Source: CAD feature listing. Evaluate the final solid. Frame: model axes, mm. Give positions to 0.01 mm unless a question says otherwise; leave off trailing zeros. Order: outer loops, then holes, each group sorted by start corner. A loop starts at its lowest first (then second) coordinate and runs counter-clockwise, first axis right, second up. Notation, with made-up numbers: M 43.5,54.25 L 92.5,54.25 A9 ccw 92.5,58.25 Z; hole C 85,9.5 d11. An arc over 180 degrees is marked long. Use CSV: the item, a comma, the result in double quotes. Start each with the question number.
Item 1: Ray query, probe 1 along X at (y, z) = (-67, -0.4); probe 2 along Y at (x, z) = (-59.5, -1.8); probe 3 along X at (y, z) = (51, -2.95). Return the intervals inside material, ascending. Write a range as from..to.
Item 2: Pull-direction query (Y, two-part tool) for faces 1 (the face through (41.116, 97.255, -1.61)), 2 (the face through (-45.549, 97.255, -1.61)), 3 (the face through (-1, 2, -3.175)); classes: +Y half, -Y half, draft (parallel to the pull), parting line (faces both ways), or undercut.
Item 3: First-contact query: pin 1 (4 mm diameter, centred on x = 59.69, y = 52.51, fed in from -Z); pin 2 (6 mm diameter, centred on x = 43.33, y = 96.96, fed in from -Z) (3 decimals). Flat tips, straight axial feed; report the tip coordinate or a pass-through.
Item 4: Section query C-C on z = -1.25. Count the separate pieces of the cut face and the enclosed holes in it, and give its area (3 significant figures).
Item 5: Section query B-B on y = -68. Return loops of the section in (x, z) (3 decimals).
Item 6: Section query A-A on x = 31.75. Return loops of the section in (y, z) (1 decimal), and give its area (3 significant figures).
Autodesk Inventor part; units mm, degrees
ref_plane "YZ Plane" through (0, 0, 0) normal (1, 0, 0) x (0, 1, 0)
ref_plane "XZ Plane" through (0, 0, 0) normal (0, 1, 0) x (-1, 0, 0)
ref_plane "XY Plane" through (0, 0, 0) normal (0, 0, 1) x (1, 0, 0)
sketch "Sketch1" plane through (0, 0, 0) normal (0, 0, 1) x (1, 0, 0)
  line L0 (-68.58, -128.7145) -> (68.58, -128.7145)
  line L1 (68.58, -128.7145) -> (68.58, 128.7145)
  line L2 (68.58, 128.7145) -> (-68.58, 128.7145)
  line L3 (-68.58, 128.7145) -> (-68.58, -128.7145)
  line L4 (-68.58, -128.7145) -> (68.58, 128.7145) construction
  line L5 (68.58, -128.7145) -> (-68.58, 128.7145) construction
  point P0 (0, 0)
  dimension "d0" = 137.16
  dimension "d1" = 257.429
extrude "Extrusion1" add sketch "Sketch1" against normal blind 3.175
sketch "Sketch2" plane through (0, 0, 0) normal (0, 0, 1) x (1, 0, 0)
  circle A0 centre (-59.69, 52.5145) radius 2.0955
  line L0 (-68.58, 128.7145) -> (-68.58, -128.7145)
  line L1 (-68.58, 128.7145) -> (68.58, 128.7145)
  circle A1 centre (59.69, 52.5145) radius 2.0955
  line L2 (68.58, -128.7145) -> (68.58, 128.7145)
  circle A2 centre (-59.69, -116.0145) radius 2.0955
  circle A3 centre (59.69, -116.0145) radius 2.0955
  line L3 (-68.58, -128.7145) -> (68.58, -128.7145)
  point P0 (0, 0)
  dimension "d4" = 8.89
  dimension "d5" = 76.2
  dimension "d6" = 76.2
  dimension "d7" = 8.89
  dimension "d8" = 4.191
  dimension "d9" = 12.7
  dimension "d10" = 8.89
  dimension "d11" = 8.89
  dimension "d12" = 12.7
  dimension "d13" = 4.191
  dimension "d21" = 4.191
  dimension "d22" = 4.191
hole "Hole1" at (-59.69, 52.5145, 0) at (59.69, 52.5145, 0) at (-59.69, -116.0145, 0) at (59.69, -116.0145, 0) direction (0, 0, -1) diameter 4.191 end through all
sketch "Sketch4" plane through (0, 0, 0) normal (0, 0, 1) x (1, 0, 0)
  line L0 (-35.179, -49.0855) -> (-35.179, -99.8855)
  line L1 (-28.321, -49.0855) -> (-28.321, -99.8855)
  line L2 (28.321, -49.0855) -> (28.321, -99.8855)
  line L3 (35.179, -49.0855) -> (35.179, -99.8855)
  line L4 (-68.58, 128.7145) -> (-68.58, -128.7145)
  line L5 (68.58, -128.7145) -> (68.58, 128.7145)
  line L6 (-68.58, -128.7145) -> (68.58, -128.7145)
  arc A0 (-28.321, -49.0855) -> (-35.179, -49.0855) centre (-31.75, -49.0855) ccw
  arc A1 (-35.179, -99.8855) -> (-28.321, -99.8855) centre (-31.75, -99.8855) ccw
  arc A2 (35.179, -49.0855) -> (28.321, -49.0855) centre (31.75, -49.0855) ccw
  arc A3 (28.321, -99.8855) -> (35.179, -99.8855) centre (31.75, -99.8855) ccw
  point P0 (0, 0)
  dimension "d23" = 6.858
  dimension "d24" = 6.858
  dimension "d25" = 33.401
  dimension "d26" = 50.8
  dimension "d27" = 33.401
  dimension "d28" = 28.829
  dimension "d29" = 28.829
  dimension "d30" = 28.829
  dimension "d31" = 28.829
  dimension "d32" = 50.8
  dimension "d33" = 50.8
  dimension "d34" = 50.8
extrude "Extrusion2" cut sketch "Sketch4" against normal blind 3.175
sketch "Sketch5" plane through (0, 0, 0) normal (0, 0, 1) x (1, 0, 0)
  line L0 (-68.58, 128.7145) -> (68.58, 128.7145)
  line L1 (68.58, 128.7145) -> (68.58, -128.7145)
  point P0 (0, 0)
  point P1 (-43.3324, 96.9645)
  point P2 (43.3324, 96.9645)
  dimension "d37" = 31.75
  dimension "d38" = 86.6648
  dimension "d39" = 31.75
  dimension "d40" = 25.2476
hole "Hole2" at (-43.3324, 96.9645, 0) at (43.3324, 96.9645, 0) direction (0, 0, -1) diameter 4.4704 end through all
sketch "smartsensorPowered" plane through (0, 0, 0) normal (0, 0, 1) x (1, 0, 0)
  line L0 (-68.58, 128.7145) -> (-68.58, -128.7145)
  line L1 (68.58, 128.7145) -> (-68.58, 128.7145)
  line L2 (68.58, -128.7145) -> (68.58, 128.7145)
  line L3 (-44.45, 33.4645) -> (-16.51, 33.4645)
  line L4 (-16.51, 33.4645) -> (-16.51, -26.2255)
  line L5 (-16.51, -26.2255) -> (-44.45, -26.2255)
  line L6 (-44.45, -26.2255) -> (-44.45, 33.4645)
  circle A0 centre (-41.275, 30.2895) radius 1.651
  circle A1 centre (-40.64, -22.4155) radius 1.651
  circle A2 centre (-19.685, 2.9845) radius 1.651
  circle A3 centre (-19.685, 30.2895) radius 1.651
  line L7 (-3.81, 33.4645) -> (24.13, 33.4645)
  line L8 (24.13, 33.4645) -> (24.13, -26.2255)
  line L9 (24.13, -26.2255) -> (-3.81, -26.2255)
  line L10 (-3.81, -26.2255) -> (-3.81, 33.4645)
  circle A4 centre (-0.635, 30.2895) radius 1.651
  circle A5 centre (0, -22.4155) radius 1.651
  circle A6 centre (20.955, 2.9845) radius 1.651
  circle A7 centre (20.955, 30.2895) radius 1.651
  point P0 (0, 0)
  dimension "d52" = 27.94
  dimension "d53" = 59.69
  dimension "d59" = 3.175
  dimension "d60" = 3.175
  dimension "d61" = 3.302
  dimension "d62" = 3.302
  dimension "d63" = 3.175
  dimension "d64" = 3.175
  dimension "d66" = 3.81
  dimension "d67" = 3.81
  dimension "d68" = 3.302
  dimension "d69" = 30.48
  dimension "d70" = 3.175
  dimension "d71" = 3.302
  dimension "d72" = 27.94
  dimension "d73" = 59.69
  dimension "d74" = 3.175
  dimension "d75" = 3.175
  dimension "d76" = 3.302
  dimension "d77" = 3.302
  dimension "d78" = 3.175
  dimension "d79" = 3.175
  dimension "d80" = 3.81
  dimension "d81" = 3.81
  dimension "d82" = 3.302
  dimension "d83" = 30.48
  dimension "d84" = 3.175
  dimension "d85" = 3.302
  dimension "d86" = 12.7
sketch "BoardArea" plane through (0, 0, 0) normal (0, 0, 1) x (1, 0, 0)
  line L0 (-50.8, 39.8145) -> (50.8, 39.8145)
  line L1 (50.8, 39.8145) -> (50.8, -36.3855)
  line L2 (50.8, -36.3855) -> (-50.8, -36.3855)
  line L3 (-50.8, -36.3855) -> (-50.8, 39.8145)
  point P0 (0, 0)
sketch "teamflag" plane through (0, 0, 0) normal (0, 0, 1) x (1, 0, 0)
  line L0 (-3.81, -7.1755) -> (-44.45, -7.1755)
  line L1 (-44.45, -7.1755) -> (-44.45, 33.4645)
  line L2 (-44.45, 33.4645) -> (-3.81, 33.4645)
  line L3 (-3.81, 33.4645) -> (-3.81, -7.1755)
  circle A0 centre (-6.35, 30.9245) radius 1.651
  circle A1 centre (-41.91, 30.9245) radius 1.651
  circle A2 centre (-41.91, -4.6355) radius 1.651
  circle A3 centre (-6.35, -4.6355) radius 1.651
  line L4 (-50.8, -36.3855) -> (-50.8, 39.8145)
  circle A4 centre (-43.3324, 96.9645) radius 2.2352
  circle A5 centre (43.3324, 96.9645) radius 2.2352
  arc A6 (-35.179, -99.8855) -> (-28.321, -99.8855) centre (-31.75, -99.8855) ccw
  line L5 (-28.321, -99.8855) -> (-28.321, -49.0855)
  arc A7 (-28.321, -49.0855) -> (-35.179, -49.0855) centre (-31.75, -49.0855) ccw
  line L6 (-35.179, -49.0855) -> (-35.179, -99.8855)
  arc A8 (28.321, -99.8855) -> (35.179, -99.8855) centre (31.75, -99.8855) ccw
  line L7 (35.179, -99.8855) -> (35.179, -49.0855)
  arc A9 (35.179, -49.0855) -> (28.321, -49.0855) centre (31.75, -49.0855) ccw
  line L8 (28.321, -49.0855) -> (28.321, -99.8855)
  circle A10 centre (-59.69, -116.0145) radius 2.0955
  circle A11 centre (-59.69, 52.5145) radius 2.0955
  circle A12 centre (59.69, 52.5145) radius 2.0955
  circle A13 centre (59.69, -116.0145) radius 2.0955
  line L9 (68.58, 128.7145) -> (68.58, -128.7145)
  line L10 (68.58, -128.7145) -> (-68.58, -128.7145)
  line L11 (-68.58, -128.7145) -> (-68.58, 128.7145)
  line L12 (-68.58, 128.7145) -> (68.58, 128.7145)
  circle A14 centre (-43.3324, 96.9645) radius 2.2352
  circle A15 centre (43.3324, 96.9645) radius 2.2352
  arc A16 (-35.179, -99.8855) -> (-28.321, -99.8855) centre (-31.75, -99.8855) ccw
  line L13 (-28.321, -99.8855) -> (-28.321, -49.0855)
  arc A17 (-28.321, -49.0855) -> (-35.179, -49.0855) centre (-31.75, -49.0855) ccw
  line L14 (-35.179, -49.0855) -> (-35.179, -99.8855)
  arc A18 (28.321, -99.8855) -> (35.179, -99.8855) centre (31.75, -99.8855) ccw
  line L15 (35.179, -99.8855) -> (35.179, -49.0855)
  arc A19 (35.179, -49.0855) -> (28.321, -49.0855) centre (31.75, -49.0855) ccw
  line L16 (28.321, -49.0855) -> (28.321, -99.8855)
  circle A20 centre (-59.69, -116.0145) radius 2.0955
  circle A21 centre (-59.69, 52.5145) radius 2.0955
  circle A22 centre (59.69, 52.5145) radius 2.0955
  circle A23 centre (59.69, -116.0145) radius 2.0955
  line L17 (68.58, 128.7145) -> (68.58, -128.7145)
  line L18 (68.58, -128.7145) -> (-68.58, -128.7145)
  line L19 (-68.58, -128.7145) -> (-68.58, 128.7145)
  line L20 (-68.58, 128.7145) -> (68.58, 128.7145)
  circle A24 centre (-43.3324, 96.9645) radius 2.2352
  circle A25 centre (43.3324, 96.9645) radius 2.2352
  arc A26 (-35.179, -99.8855) -> (-28.321, -99.8855) centre (-31.75, -99.8855) ccw
  line L21 (-28.321, -99.8855) -> (-28.321, -49.0855)
  arc A27 (-28.321, -49.0855) -> (-35.179, -49.0855) centre (-31.75, -49.0855) ccw
  line L22 (-35.179, -49.0855) -> (-35.179, -99.8855)
  arc A28 (28.321, -99.8855) -> (35.179, -99.8855) centre (31.75, -99.8855) ccw
  line L23 (35.179, -99.8855) -> (35.179, -49.0855)
  arc A29 (35.179, -49.0855) -> (28.321, -49.0855) centre (31.75, -49.0855) ccw
  line L24 (28.321, -49.0855) -> (28.321, -99.8855)
  circle A30 centre (-59.69, -116.0145) radius 2.0955
  circle A31 centre (-59.69, 52.5145) radius 2.0955
  circle A32 centre (59.69, 52.5145) radius 2.0955
  circle A33 centre (59.69, -116.0145) radius 2.0955
  line L25 (68.58, 128.7145) -> (68.58, -128.7145)
  line L26 (68.58, -128.7145) -> (-68.58, -128.7145)
  line L27 (-68.58, -128.7145) -> (-68.58, 128.7145)
  line L28 (-68.58, 128.7145) -> (68.58, 128.7145)
  circle A34 centre (-43.3324, 96.9645) radius 2.2352
  circle A35 centre (43.3324, 96.9645) radius 2.2352
  arc A36 (-35.179, -99.8855) -> (-28.321, -99.8855) centre (-31.75, -99.8855) ccw
  line L29 (-28.321, -99.8855) -> (-28.321, -49.0855)
  arc A37 (-28.321, -49.0855) -> (-35.179, -49.0855) centre (-31.75, -49.0855) ccw
  line L30 (-35.179, -49.0855) -> (-35.179, -99.8855)
  arc A38 (28.321, -99.8855) -> (35.179, -99.8855) centre (31.75, -99.8855) ccw
  line L31 (35.179, -99.8855) -> (35.179, -49.0855)
  arc A39 (35.179, -49.0855) -> (28.321, -49.0855) centre (31.75, -49.0855) ccw
  line L32 (28.321, -49.0855) -> (28.321, -99.8855)
  circle A40 centre (-59.69, -116.0145) radius 2.0955
  circle A41 centre (-59.69, 52.5145) radius 2.0955
  circle A42 centre (59.69, 52.5145) radius 2.0955
  circle A43 centre (59.69, -116.0145) radius 2.0955
  line L33 (68.58, 128.7145) -> (68.58, -128.7145)
  line L34 (68.58, -128.7145) -> (-68.58, -128.7145)
  line L35 (-68.58, -128.7145) -> (-68.58, 128.7145)
  line L36 (-68.58, 128.7145) -> (68.58, 128.7145)
  circle A44 centre (-43.3324, 96.9645) radius 2.2352
  circle A45 centre (43.3324, 96.9645) radius 2.2352
  arc A46 (-35.179, -99.8855) -> (-28.321, -99.8855) centre (-31.75, -99.8855) ccw
  line L37 (-28.321, -99.8855) -> (-28.321, -49.0855)
  arc A47 (-28.321, -49.0855) -> (-35.179, -49.0855) centre (-31.75, -49.0855) ccw
  line L38 (-35.179, -49.0855) -> (-35.179, -99.8855)
  arc A48 (28.321, -99.8855) -> (35.179, -99.8855) centre (31.75, -99.8855) ccw
  line L39 (35.179, -99.8855) -> (35.179, -49.0855)
  arc A49 (35.179, -49.0855) -> (28.321, -49.0855) centre (31.75, -49.0855) ccw
  line L40 (28.321, -49.0855) -> (28.321, -99.8855)
  circle A50 centre (-59.69, -116.0145) radius 2.0955
  circle A51 centre (-59.69, 52.5145) radius 2.0955
  circle A52 centre (59.69, 52.5145) radius 2.0955
  circle A53 centre (59.69, -116.0145) radius 2.0955
  line L41 (68.58, 128.7145) -> (68.58, -128.7145)
  line L42 (68.58, -128.7145) -> (-68.58, -128.7145)
  line L43 (-68.58, -128.7145) -> (-68.58, 128.7145)
  line L44 (-68.58, 128.7145) -> (68.58, 128.7145)
  line L45 (-50.8, 39.8145) -> (50.8, 39.8145)
  line L46 (43.18, -7.1755) -> (2.54, -7.1755)
  line L47 (2.54, -7.1755) -> (2.54, 33.4645)
  line L48 (2.54, 33.4645) -> (43.18, 33.4645)
  line L49 (43.18, 33.4645) -> (43.18, -7.1755)
  circle A54 centre (40.64, 30.9245) radius 1.651
  circle A55 centre (5.08, 30.9245) radius 1.651
  circle A56 centre (5.08, -4.6355) radius 1.651
  circle A57 centre (40.64, -4.6355) radius 1.651
  dimension "d100" = 3.302
  dimension "d101" = 40.64
  dimension "d102" = 40.64
  dimension "d103" = 2.54
  dimension "d104" = 2.54
  dimension "d105" = 2.54
  dimension "d106" = 38.1
  dimension "d107" = 38.1
  dimension "d108" = 2.54
  dimension "d109" = 38.1
  dimension "d110" = 38.1
  dimension "d113" = 3.302
  dimension "d114" = 40.64
  dimension "d115" = 40.64
  dimension "d116" = 2.54
  dimension "d117" = 2.54
  dimension "d118" = 2.54
  dimension "d119" = 38.1
  dimension "d120" = 38.1
  dimension "d121" = 2.54
  dimension "d122" = 38.1
  dimension "d123" = 38.1
  dimension "d124" = 6.35
sketch "cape" plane through (0, 0, 0) normal (0, 0, 1) x (1, 0, 0)
  line L0 (-44.45, -21.1355) -> (27.61, -21.1355)
  line L1 (27.61, -21.1355) -> (27.61, 33.4645)
  line L2 (27.61, 33.4645) -> (-44.45, 33.4645)
  line L3 (-44.45, 33.4645) -> (-44.45, -21.1355)
  circle A0 centre (-41.275, -17.9605) radius 1.5875
  circle A1 centre (24.765, -14.7855) radius 1.5875
  circle A2 centre (24.765, 27.1245) radius 1.5875
  circle A3 centre (-41.275, 30.2995) radius 1.5875
  line L4 (-50.8, 39.8145) -> (50.8, 39.8145)
  line L5 (-50.8, -36.3855) -> (-50.8, 39.8145)
  point P0 (0, 0)
  dimension "d125" = 3.175
  dimension "d126" = 72.06
  dimension "d127" = 54.6
  dimension "d130" = 2.845
  dimension "d131" = 6.34
  dimension "d132" = 2.845
  dimension "d133" = 48.25
  dimension "d134" = 68.885
  dimension "d135" = 3.165
  dimension "d136" = 68.885
  dimension "d137" = 51.425
Verdict:
1,probe 1,"-68.58..-35.18, -28.32..28.32, 35.18..68.58"
1,probe 2,"-128.71..-118.1, -113.93..50.43, 54.6..128.71"
1,probe 3,"-68.58..-61.14, -58.24..58.24, 61.14..68.58"
2,face 1,"undercut"
2,face 2,"undercut"
2,face 3,"draft"
3,pin 1,"through"
3,pin 2,"z = -3.175"
4,separate pieces,"1"
4,enclosed holes,"8"
4,area,"34,500 mm2"
5,outline,"M -68.58,-3.175 L -35.179,-3.175 L -35.179,0 L -68.58,0 Z; M -28.321,-3.175 L 28.321,-3.175 L 28.321,0 L -28.321,0 Z; M 35.179,-3.175 L 68.58,-3.175 L 68.58,0 L 35.179,0 Z"
6,outline,"M -128.7,-3.2 L -103.3,-3.2 L -103.3,0 L -128.7,0 Z; M -45.7,-3.2 L 128.7,-3.2 L 128.7,0 L -45.7,0 Z"
6,area,"634 mm2"
